Build history of the part. All positions in model axes, mm. A direction names the side the tool comes from. Give positions to 0.01 mm unless a question says otherwise; leave off trailing zeros. Order: outer loops, then holes, each group sorted by start corner. A loop starts at its lowest first (then second) coordinate and runs counter-clockwise, first axis right, second up. Notation, with made-up numbers: (43, 77.25) - (79, 77.25) arc R7 ccw to (79, 82.25) - close; hole circle Ø4 at (-13, -32.5). An arc over 180 degrees is marked (long way). Answer in a Markdown table with one row per item.
Autodesk Inventor part; units mm, degrees
ref_plane "bgrrb_to_rring_XY" through (9, 0, 0) normal (1, 0, 0) x (0, 0, -1)
ref_plane "bgrrb_to_rring_YZ" through (9, 0, 0) normal (0, 0, -1) x (0, 1, 0)
ref_plane "bgrrb_to_rring_ZX" through (9, 0, 0) normal (0, 1, 0) x (1, 0, 0)
sketch "Sketch_1" plane through (0, 0, 0) normal (1, 0, 0) x (0, 1, 0)
  circle A0 centre (0, 0) radius 22.5
extrude "Extrusion1" add sketch "Sketch_1" along normal blind 12
sketch "Sketch_2" plane through (0, 0, 0) normal (0, 0, 1) x (1, 0, 0)
  line L0 (12, 0) -> (0, 0)
  line L1 (0, 0) -> (0, 9)
  line L2 (0, 9) -> (2, 9)
  line L3 (2, 9) -> (2, 11)
  line L4 (2, 11) -> (9, 11)
  line L5 (9, 11) -> (9, 11.75)
  line L6 (9, 11.75) -> (10.15, 11.75)
  line L7 (10.15, 11.75) -> (10.15, 11)
  line L8 (10.15, 11) -> (12, 11)
  line L9 (12, 11) -> (12, 0)
  line L10 (12, 0) -> (0, 0)
revolve "Revolution1" cut sketch "Sketch_2" angle 360 about axis through (12, 0, 0) along (1, 0, 0)
sketch "Sketch_9" plane through (0, 0, 0) normal (0, 0, 1) x (1, 0, 0)
  line L0 (12, 17.5) -> (2, 17.5)
  line L1 (2, 17.5) -> (2, 20)
  line L2 (2, 20) -> (2.433, 19.567)
  line L3 (2.433, 19.567) -> (7.167, 19.567)
  line L4 (7.167, 19.567) -> (7.6, 20)
  line L5 (7.6, 20) -> (7.6, 21.5)
  line L6 (7.6, 21.5) -> (12, 21.5)
  line L7 (12, 21.5) -> (12, 17.5)
  line L8 (12, 17.5) -> (2, 17.5)
revolve "Revolution2" cut sketch "Sketch_9" angle 360 about axis through (12, 17.5, 0) along (1, 0, 0)
thread "Thread1"
sketch "Sketch_4" plane through (0, 0, 0) normal (1, 0, 0) x (0, 1, 0)
  circle A0 centre (0, 0) radius 46
  circle A1 centre (0, 0) radius 13.5
extrude "Extrusion2" cut sketch "Sketch_4" along normal blind 2
pattern_linear "Rectangular Pattern1" count 2 spacing 24.7487 along (0, -0.7071, 0.7071) count 2 spacing 24.7487 along (0, -0.7071, -0.7071) of "Revolution2"
ref_plane "bgrrb_to_rring_XY" through (9, 0, 0) normal (1, 0, 0) x (0, 0, -1)
ref_plane "bgrrb_to_rring_YZ" through (9, 0, 0) normal (0, 0, -1) x (0, 1, 0)
ref_plane "bgrrb_to_rring_ZX" through (9, 0, 0) normal (0, 1, 0) x (1, 0, 0)
ref_plane "housing_to_dummy_XY" through (0, 0, 0) normal (0, 0, 1) x (1, 0, 0)
ref_plane "housing_to_dummy_YZ" through (0, 0, 0) normal (1, 0, 0) x (0, 1, 0)
ref_plane "housing_to_dummy_ZX" through (0, 0, 0) normal (0, 1, 0) x (0, 0, 1)
ref_plane "to_bearings_1_XY" through (2, 0, 0) normal (1, 0, 0) x (0, 0, -1)
ref_plane "to_bearings_1_YZ" through (2, 0, 0) normal (0, 0, -1) x (0, 1, 0)
ref_plane "to_bearings_1_ZX" through (2, 0, 0) normal (0, 1, 0) x (1, 0, 0)
properties part number "BARR608ZZ_b"
1. Cut at A-A on y = -8. Write the cut outline in (x, z).
Check result:
| item | result |
|---|---|
| outline | (0, -10.87) - (2, -10.87) - (2, -21.03) - (12, -21.03) - (12, -7.55) - (10.15, -7.55) - (10.15, -8.61) - (9, -8.61) - (9, -7.55) - (2, -7.55) - (2, -4.12) - (0, -4.12) - close; (0, 4.12) - (2, 4.12) - (2, 7.55) - (9, 7.55) - (9, 8.61) - (10.15, 8.61) - (10.15, 7.55) - (12, 7.55) - (12, 21.03) - (2, 21.03) - (2, 10.87) - (0, 10.87) - close |
2. Drop flat-ended pins along their axis: P1, Ø5, axis at y = 5, z = 16, coming from the -X side; P2, Ø4, axis at x = 5, z = 7, coming from the +Y side; P3, Ø4, axis at y = 18, z = 1, coming from the +X side. Give the stop position or say it passes through.
Check result:
| item | result |
|---|---|
| P1 | stops at x = 2 |
| P2 | stops at y = 21.94 |
| P3 | stops at x = 7.6 |
3. Which spindle directions (+Z, -Z, +X, -X, +Y, -Y) get a long thin tool onto all of the face, cutting with end or side? Do faces 1 (the face through (9.583, 11.207, 3.529)), 2 (the face through (4.83, 19.47, 0.62)), 3 (the face through (9.831, 13.504, 0.176)). Say none if no direction does.
Check result:
| item | result |
|---|---|
| face 1 | none |
| face 2 | +X, -X |
| face 3 | +X |
4. Probe line 1 (X direction, y = 0.5, z = -11.5); line 2 (Y direction, x = 11.75, z = 3.5); line 3 (Y direction, x = 8, z = -0.5). List the from-to ranges inside material, lowest first.
Check result:
| item | result |
|---|---|
| line 1 | x = 0 to 9, 10.15 to 12 |
| line 2 | y = -22.23 to -19.44, -15.56 to -10.43, 10.43 to 15.56, 19.44 to 22.23 |
| line 3 | y = -22.49 to -21.47, -13.53 to -10.99, 10.99 to 13.53, 21.47 to 22.49 |
5. Two-plate mould, pull along Y, no slides. Class faces 4 (the face through (9.831, -0.867, -21.405)), 5 (the face through (2, 10, -10)): +Y half, -Y half, draft (parallel to the pull), parting line (faces both ways), or undercut.
Check result:
| item | result |
|---|---|
| face 4 | undercut |
| face 5 | draft |
6. Cut at B-B on z = 0. Count the separate pieces of the cut face and the enclosed holes in it, and give its area (3 significant figures).
Check result:
| item | result |
|---|---|
| separate pieces | 4 |
| enclosed holes | 0 |
| area | 129 mm² |
